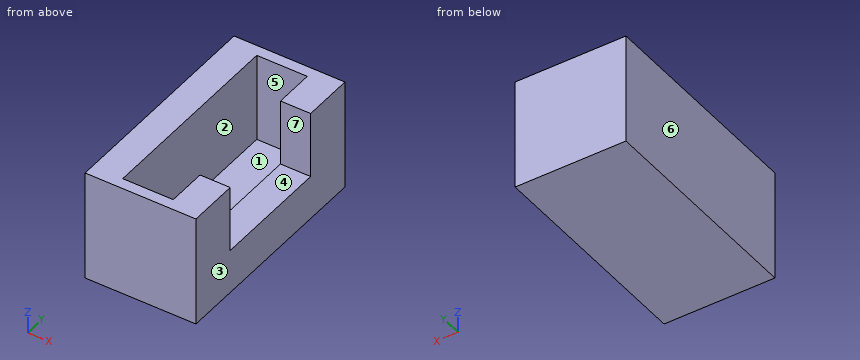
from build123d import *

# Parameters (mm, degrees)
F0_W     = 10
F0_H     = 20
F1_DEPTH = 10
F3_DEPTH = 8
F2_W     = 2.72019
F2_H     = 10.8
F4_DEPTH = 6


with BuildPart() as f1:
    # F0 (on Top) → F1 (new body)
    with BuildSketch(Plane.XY):
        Rectangle(F0_W, F0_H)
    extrude(amount=F1_DEPTH)

    # F2 (on face) → F3 (cut)
    with BuildSketch(Plane.XY.offset(10)):
        Polygon((2.27981, 5.4), (2.27981, 9), (-2.27981, 9), (-2.27981, -9), (2.27981, -9), (2.27981, -5.4), align=None)
    extrude(amount=-F3_DEPTH, mode=Mode.SUBTRACT)

    # F2 (on face) → F4 (cut)
    with BuildSketch(Plane.XY.offset(10)):
        with Locations((3.639905, 0)):
            Rectangle(F2_W, F2_H)
    extrude(amount=-F4_DEPTH, mode=Mode.SUBTRACT)


solid = f1.part
The model under review builds one solid part; all positions refer to its coordinate system, in mm. Face numbers are marked on the shaded views. A direction names the side the tool comes from. Round coordinates to 2 decimals unless told otherwise and drop trailing zeros. Loops run counter-clockwise (first coordinate to the right, second up) from the corner with the lowest first, then second, coordinate; pieces in that order, holes last. Notation, with made-up numbers: (12, 25.25) -> (28, 25.25) arc R19 ccw to (28, 30.25) -> close; hole circle Ø5 at (73, 43). An arc over 180 degrees is marked (long way). Answer as CSV lines item,"result".
1) Tool access review of the marked faces 5, 6 and 7: name each direction out of +Z, -Z, +X, -X, +Y, -Y from which nothing blocks a thin tool from reaching the whole face with its end or side.
Geometry results:
face 5,"+Z"
face 6,"+Z, -Z, -X, +Y, -Y"
face 7,"+Z, +X"
2) Add section C-C on y = -2.75. Write out the cut boundary in (x, z), plus the area to 3 significant figures.
Geometry results:
outline,"(-5, 0) -> (5, 0) -> (5, 4) -> (2.28, 4) -> (2.28, 2) -> (-2.28, 2) -> (-2.28, 10) -> (-5, 10) -> close"
area,"47.2 mm²"
3) Add section D-D on z = 5. Write out the cut boundary in (x, y), plus the area to 3 significant figures.
Geometry results:
outline,"(-5, -10) -> (5, -10) -> (5, -5.4) -> (2.28, -5.4) -> (2.28, -9) -> (-2.28, -9) -> (-2.28, 9) -> (2.28, 9) -> (2.28, 5.4) -> (5, 5.4) -> (5, 10) -> (-5, 10) -> close"
area,"88.5 mm²"
4) For P1, Ø3, axis at x = 3.5, y = -1, coming from the +Z side; P2, Ø4, axis at y = 2, z = 6.5, coming from the +X side, all flat-tipped, find the tip position at first contact; note any pin that passes through.
Geometry results:
P1,"stops at z = 4"
P2,"stops at x = -2.28"
5) To check wall thickness, follow line 1 along Y through (x, z) = (3.5, 7.25); line 2 along X through (y, z) = (-7.5, 3.25); line 3 along Y through (x, z) = (-1, 2.5). State the ranges of each line that lie inside material, in increasing order. Write a range as from..to.
Geometry results:
line 1,"y = -10..-5.4, 5.4..10"
line 2,"x = -5..-2.28, 2.28..5"
line 3,"y = -10..-9, 9..10"
6) Draft analysis for pull direction X (two halves, no side actions). For the marked faces 1, 2, 3 and 4, state which applies: pulls with the +X half, pulls with the -X half, needs draft (parallel to the pull), parting line crosses it, or undercut.
Geometry results:
face 1,"undercut"
face 2,"undercut"
face 3,"pulls with the +X half"
face 4,"needs draft"
7) Add section B-B on x = 3.5. Write out the cut boundary in (y, z), plus the area to 3 significant figures.
Geometry results:
outline,"(-10, 0) -> (10, 0) -> (10, 10) -> (5.4, 10) -> (5.4, 4) -> (-5.4, 4) -> (-5.4, 10) -> (-10, 10) -> close"
area,"135 mm²"
8) Add section A-A on z = 2.75. Write out the cut boundary in (x, y).
Geometry results:
outline,"(-5, -10) -> (5, -10) -> (5, 10) -> (-5, 10) -> close; hole (-2.28, -9) -> (2.28, -9) -> (2.28, 9) -> (-2.28, 9) -> close"
